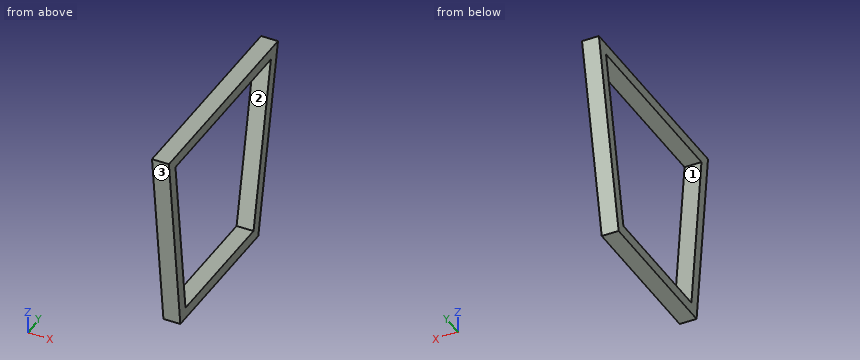
from build123d import *

# Parameters (mm, degrees)
F1_DEPTH = 30


with BuildPart() as f1:
    # F0 (on Right) → F1 (new body)
    with BuildSketch(Plane.YZ):
        Polygon((399.73456, 0), (467.591669, 334.999998), (92.28704, 334.999998), (131.5781, 0), align=None)
        Polygon((114.769867, 314.999998), (443.134323, 314.999998), (383.379555, 20), (149.369457, 20), align=None, mode=Mode.SUBTRACT)
    extrude(amount=-F1_DEPTH)


solid = f1.part
The listing builds one solid part. Answer for the finished solid, in the listing's coordinates (mm). Face numbers are marked on the shaded views. Give positions to 0.01 mm unless a question says otherwise; leave off trailing zeros. Order: outer loops, then holes, each group sorted by start corner. A loop starts at its lowest first (then second) coordinate and runs counter-clockwise, first axis right, second up. Notation, with made-up numbers: (9, 80.5) - (43, 80.5) arc R6 cw to (43, 91.5) - close; hole circle Ø4 at (84.5, -24). An arc over 180 degrees is marked (long way). Answer as CSV lines item,"result".
Q1. Straight lines are drawn through the part: L1, parallel to Z at x = -6, y = 222; L2, parallel to Y at x = -3, z = 43; L3, parallel to Y at x = -28.5, z = 85. For each, find the intervals that lie inside material, in ascending order.
Answer key:
L1,"z = 0 to 20, 315 to 335"
L2,"y = 126.53 to 146.67, 388.04 to 408.44"
L3,"y = 121.61 to 141.75, 396.55 to 416.95"
Q2. A cutting plane is placed at C-C, the plane z = 30. Determine the outline of the cut face in (x, y), and give its area (3 significant figures).
Answer key:
outline,"(-30, 128.06) - (0, 128.06) - (0, 148.2) - (-30, 148.2) - close; (-30, 385.41) - (0, 385.41) - (0, 405.81) - (-30, 405.81) - close"
area,"1,220 mm^2"
Q3. Determine the mould class of the marked faces 1, 2 and 3 for opening direction Z: pulls with the +Z half, pulls with the -Z half, needs draft (parallel to the pull), parting line crosses it, or undercut.
Answer key:
face 1,"undercut"
face 2,"undercut"
face 3,"pulls with the -Z half"
Q4. A cutting plane is placed at A-A, the plane x = -10.25. Determine the outline of the cut face in (y, z).
Answer key:
outline,"(92.29, 335) - (131.58, 0) - (399.73, 0) - (467.59, 335) - close; hole (114.77, 315) - (149.37, 20) - (383.38, 20) - (443.13, 315) - close"
Q5. A cutting plane is placed at B-B, the plane y = 340.5. Determine the outline of the cut face in (x, z).
Answer key:
outline,"(-30, 0) - (0, 0) - (0, 20) - (-30, 20) - close; (-30, 315) - (0, 315) - (0, 335) - (-30, 335) - close"
Q6. Each of these flat-tipped pins is pushed along its axis until it touches: pin 1 Ø1 at (x, z) = (-24, 88.5) entering from -Y; pin 2 Ø1 at (x, z) = (-20, 243.5) entering from -Y; pin 3 Ø6 at (x, z) = (-21, 90) entering from -Y. Where does it stop, or does it pass through?
Answer key:
pin 1,"stops at y = 121.14"
pin 2,"stops at y = 102.96"
pin 3,"stops at y = 120.67"
